Geometry check sheet. Reference: the model listing, model coordinates, mm. Face numbers are marked on the shaded views. Round coordinates to 2 decimals unless told otherwise and drop trailing zeros. Write each loop counter-clockwise with the first axis right and the second up, starting at its lowest first coordinate (ties: lowest second). Pieces come first, ordered by that corner, then holes.
Item 1: Cross-section at C-C (y = 223). Enter the section's corners in (x, z).
Item 2: Cross-section at A-A (x = 0). Enter the section's corners in (y, z).
Item 3: Scan lines: probe 1 along X at (y, z) = (6.5, -24); probe 2 along X at (y, z) = (127.5, 0). Record each from-to range of solid material in increasing order.
Item 4: Cross-section at B-B (z = 0). Enter the section's corners in (x, y), then the cut area to 3 significant figures.
Item 5: Depth check by flat-ended pin: P1, Ø7, axis at x = -24, z = 24, coming from the +Y side; P2, Ø10, axis at y = 102, z = 8, coming from the -X side; P3, Ø5.5, axis at x = 24, z = -24, coming from the -Y side; P4, Ø3, axis at x = -5.5, y = 162.5, coming from the +Z side. Enter the tip coordinate at first touch or a pass-through.
Item 6: Draft check along Z on the marked faces 1, 2 and 3. Enter one of: pulls with the +Z half, pulls with the -Z half, needs draft (parallel to the pull), parting line crosses it, or undercut.
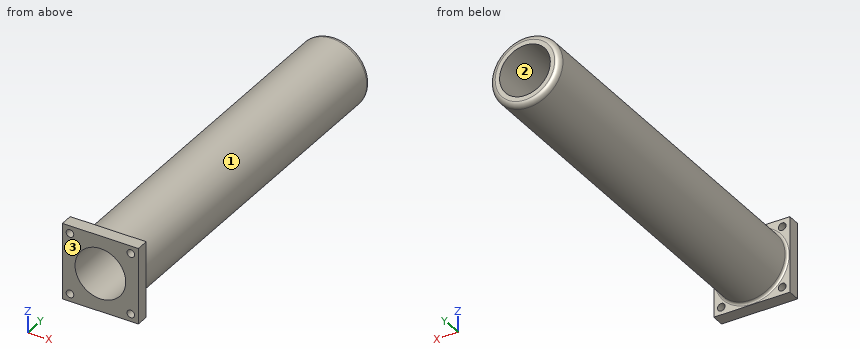
from build123d import *

# Parameters (mm, degrees)
SZKIC1_W                    = 60
SZKIC1_H                    = 60
DODANIE_WYCI_GNI_CIE1_DEPTH = 300
SZKIC2_OUTSIDE_W            = 124.354
SZKIC2_OUTSIDE_H            = 124.354
SZKIC2_OUTSIDE_R            = 27.5
WYTNIJ_WYCI_GNI_CIE1_DEPTH  = 290
SZKIC5_R                    = 20
WYTNIJ_WYCI_GNI_CIE3_DEPTH  = 303.985148151
ZAOKR_GLENIE2_R             = 2
ZAOKR_GLENIE3_R             = 4
OTWORY_USTALAJ_CE_6_0MM1_D  = 6


with BuildPart() as part:
    # Szkic1 → Dodanie-wyciągnięcie1 (new body)
    with BuildSketch(Plane(origin=(0, 0, 0), x_dir=(1, 0, 0), z_dir=(0, 1, 0))):
        Rectangle(SZKIC1_W, SZKIC1_H)
    extrude(amount=DODANIE_WYCI_GNI_CIE1_DEPTH)

    # Szkic2 outside → Wytnij-wyciągnięcie1 (cut)
    with BuildSketch(Plane(origin=(0, 300, 0), x_dir=(1, 0, 0), z_dir=(0, 1, 0))):
        Rectangle(SZKIC2_OUTSIDE_W, SZKIC2_OUTSIDE_H)
        with Locations(Location((0, 0, 0), (0, 0, 270))):
            Circle(SZKIC2_OUTSIDE_R, mode=Mode.SUBTRACT)
    extrude(amount=-WYTNIJ_WYCI_GNI_CIE1_DEPTH, mode=Mode.SUBTRACT)

    # Szkic5 → Wytnij-wyciągnięcie3 (cut, through all)
    with BuildSketch(Plane(origin=(0, 300, 0), x_dir=(1, 0, 0), z_dir=(0, 1, 0))):
        with Locations(Location((0, 0, 0), (0, 0, 270))):
            Circle(SZKIC5_R)
    extrude(amount=-WYTNIJ_WYCI_GNI_CIE3_DEPTH, mode=Mode.SUBTRACT)

    # Zaokrąglenie2
    zaokr_glenie2_edges = [part.edges().sort_by_distance(p)[0] for p in [
        (0, 10, -27.5),
    ]]
    fillet(zaokr_glenie2_edges, radius=ZAOKR_GLENIE2_R)

    # Zaokrąglenie3
    zaokr_glenie3_edges = [part.edges().sort_by_distance(p)[0] for p in [
        (0, 300, -27.5),
    ]]
    fillet(zaokr_glenie3_edges, radius=ZAOKR_GLENIE3_R)

    # Otwory ustalające Ø6.0mm1 (through all)
    with Locations(Plane(origin=(0, 10, 0), x_dir=(1, 0, 0), z_dir=(0, 1, 0))):
        with Locations((-24, -24), (-24, 24), (24, 24), (24, -24)):
            Hole(OTWORY_USTALAJ_CE_6_0MM1_D / 2)


solid = part.part
Resolved:
1. outline: circle Ø55 at (0, 0); hole circle Ø40 at (0, 0)
2. outline: (0, -30) - (10, -30) - (10, -29.5) arc R2 cw to (12, -27.5) - (296, -27.5) arc R4 ccw to (300, -23.5) - (300, -20) - (0, -20) - close; (0, 20) - (300, 20) - (300, 23.5) arc R4 ccw to (296, 27.5) - (12, 27.5) arc R2 cw to (10, 29.5) - (10, 30) - (0, 30) - close
3. probe 1: x = -30 to -27, -21 to 21, 27 to 30
3. probe 2: x = -27.5 to -20, 20 to 27.5
4. outline: (-30, 0) - (-20, 0) - (-20, 300) - (-23.5, 300) arc R4 ccw to (-27.5, 296) - (-27.5, 12) arc R2 cw to (-29.5, 10) - (-30, 10) - close; (20, 0) - (30, 0) - (30, 10) - (29.5, 10) arc R2 cw to (27.5, 12) - (27.5, 296) arc R4 ccw to (23.5, 300) - (20, 300) - close
4. area: 4,540 mm2
5. P1: stops at y = 10
5. P2: stops at x = -27.34
5. P3: passes through
5. P4: stops at z = 27.21
6. face 1: parting line crosses it
6. face 2: undercut
6. face 3: needs draft
